Source: CAD feature listing. Evaluate the final solid. Frame: model axes, mm. Face numbers are marked on the shaded views. A direction names the side the tool comes from. Coordinates: 2 decimals unless noted, no trailing zeros. Order: outer loops, then holes, each group sorted by start corner. A loop starts at its lowest first (then second) coordinate and runs counter-clockwise, first axis right, second up. Notation, with made-up numbers: (-2.5, 29) - (3.5, 29) arc R16 cw to (3.5, 46) - close; hole circle Ø7 at (-12.5, 13). An arc over 180 degrees is marked (long way). One line per question, with ' | ' between items.
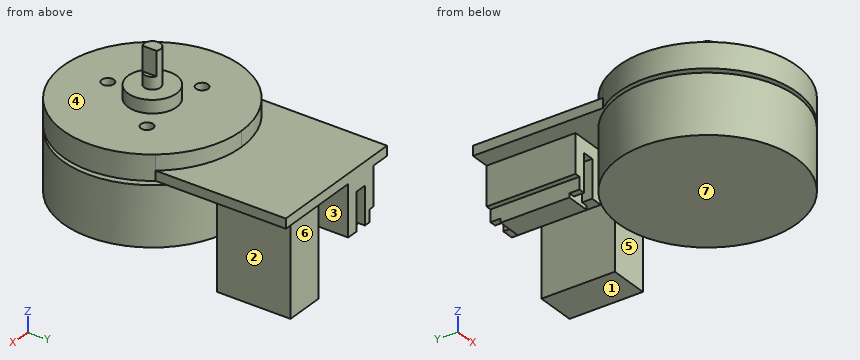
from build123d import *

# Parameters (mm, degrees)
SKETCH1_R           = 22
BOSS_EXTRUDE1_DEPTH = 21.83
SKETCH2_R           = 6
SKETCH2_R_2         = 2
BOSS_EXTRUDE2_DEPTH = 3.2
SKETCH3_R           = 2
BOSS_EXTRUDE3_DEPTH = 12.2
BOSS_EXTRUDE4_START = -6.2
BOSS_EXTRUDE4_DEPTH = 6.2
CUT_EXTRUDE3_START  = -3.8
CUT_EXTRUDE3_DEPTH  = 3.8
SKETCH7_W           = 9.7
SKETCH7_H           = 18.15
BOSS_EXTRUDE5_DEPTH = 26.4
SKETCH7_3_W         = 8.71
SKETCH7_3_H         = 22
BOSS_EXTRUDE6_DEPTH = 15
SKETCH8_R           = 1.5
CUT_EXTRUDE4_DEPTH  = 5
SKETCH9_W           = 1
SKETCH9_H           = 3.350814255
SKETCH10_W          = 6
SKETCH10_H          = 17
BOSS_EXTRUDE7_DEPTH = 1
SKETCH12_W          = 1.355
SKETCH12_H          = 22
CUT_EXTRUDE5_DEPTH  = 3
SKETCH13_W          = 2.841503492
SKETCH13_H          = 2.5
CUT_EXTRUDE6_DEPTH  = 9.35
CUT_EXTRUDE7_START  = -6
CUT_EXTRUDE7_DEPTH  = 6


with BuildPart() as part:
    # Sketch1 → Boss-Extrude1 (new body)
    with BuildSketch(Plane.XY):
        with Locations(Location((0, 0, 0), (0, 0, 180))):
            Circle(SKETCH1_R)
    extrude(amount=BOSS_EXTRUDE1_DEPTH)

    # Sketch2 → Boss-Extrude2 (add)
    with BuildSketch(Plane.XY.offset(21.83)):
        Circle(SKETCH2_R)
        Circle(SKETCH2_R_2, mode=Mode.SUBTRACT)
    extrude(amount=BOSS_EXTRUDE2_DEPTH)

    # Sketch3 → Boss-Extrude3 (add)
    with BuildSketch(Plane.XY.offset(21.83)):
        Circle(SKETCH3_R)
    extrude(amount=BOSS_EXTRUDE3_DEPTH)

    # Sketch4 → Boss-Extrude4 (add)
    with BuildSketch(Plane.XY.offset(21.83).offset(BOSS_EXTRUDE4_START)):
        Polygon((-17.5, 45.5), (-17.5, 22), (0, 22), (17.5, 22), (17.5, 45.5), align=None)
        with BuildLine():
            Line((0, 22), (-17.5, 22))
            Line((-17.5, 22), (-17.5, 13.332291626))
            ThreePointArc((-17.5, 13.332291626), (-9.764465787, 19.714340159), (0, 22))
        make_face()
        with BuildLine():
            Line((17.5, 22), (0, 22))
            ThreePointArc((0, 22), (9.764465787, 19.714340159), (17.5, 13.332291626))
            Line((17.5, 13.332291626), (17.5, 22))
        make_face()
    extrude(amount=BOSS_EXTRUDE4_DEPTH)

    # Sketch4_4 → Cut-Extrude3 (cut)
    with BuildSketch(Plane.XY.offset(21.83).offset(CUT_EXTRUDE3_START)):
        Polygon((-17.5, 45.5), (-17.5, 22), (0, 22), (17.5, 22), (17.5, 45.5), align=None)
        with BuildLine():
            Line((0, 22), (-17.5, 22))
            Line((-17.5, 22), (-17.5, 13.332291626))
            ThreePointArc((-17.5, 13.332291626), (-9.764465787, 19.714340159), (0, 22))
        make_face()
        with BuildLine():
            Line((17.5, 22), (0, 22))
            ThreePointArc((0, 22), (9.764465787, 19.714340159), (17.5, 13.332291626))
            Line((17.5, 13.332291626), (17.5, 22))
        make_face()
    extrude(amount=CUT_EXTRUDE3_DEPTH, mode=Mode.SUBTRACT)

    # Sketch7 → Boss-Extrude5 (add)
    with BuildSketch(Plane.XY.offset(18.03)):
        with Locations((8.23, 34.425)):
            Rectangle(SKETCH7_W, SKETCH7_H)
    extrude(amount=-BOSS_EXTRUDE5_DEPTH)

    # Sketch7_3 → Boss-Extrude6 (add)
    with BuildSketch(Plane.XY.offset(18.03)):
        with Locations((-8.445, 34.5)):
            Rectangle(SKETCH7_3_W, SKETCH7_3_H)
    extrude(amount=-BOSS_EXTRUDE6_DEPTH)

    # Sketch8 → Cut-Extrude4 (cut)
    with BuildSketch(Plane.XY.offset(21.83)):
        with Locations((-9.526279442, 5.5)):
            Circle(SKETCH8_R)
        with Locations((9.526279442, 5.5)):
            Circle(SKETCH8_R)
        with Locations((0, -11)):
            Circle(SKETCH8_R)
    extrude(amount=-CUT_EXTRUDE4_DEPTH, mode=Mode.SUBTRACT)

    # Sketch9 → Cut-Revolve1 (revolve, cut)
    with BuildSketch(Plane(origin=(0, 0, 0), x_dir=(0, 0, -1), z_dir=(1, 0, 0)), mode=Mode.PRIVATE) as cut_revolve1_sk:
        with Locations((-15.13, 20.324592872)):
            Rectangle(SKETCH9_W, SKETCH9_H)
    revolve(cut_revolve1_sk.sketch.rotate(Axis((0, 0, 34.03), (0, 0, -1)), 307.301790292), axis=Axis((0, 0, 34.03), (0, 0, -1)), mode=Mode.SUBTRACT)

    # Sketch10 → Boss-Extrude7 (add)
    with BuildSketch(Plane(origin=(0, 0, 3.03), x_dir=(-1, 0, 0), z_dir=(0, 0, -1))):
        with Locations((8.445, 34.5)):
            Rectangle(SKETCH10_W, SKETCH10_H)
    extrude(amount=BOSS_EXTRUDE7_DEPTH)

    # Sketch12 → Cut-Extrude5 (cut)
    with BuildSketch(Plane(origin=(0, 0, 3.03), x_dir=(-1, 0, 0), z_dir=(0, 0, -1))):
        with Locations((12.1225, 34.5)):
            Rectangle(SKETCH12_W, SKETCH12_H)
    extrude(amount=-CUT_EXTRUDE5_DEPTH, mode=Mode.SUBTRACT)

    # Sketch13 → Cut-Extrude6 (cut)
    with BuildSketch(Plane(origin=(0, 0, 3.03), x_dir=(-1, 0, 0), z_dir=(0, 0, -1))):
        with Locations((8.445, 44.25)):
            Rectangle(SKETCH13_W, SKETCH13_H)
        with Locations((8.445, 24.75)):
            Rectangle(SKETCH13_W, SKETCH13_H)
    extrude(amount=-CUT_EXTRUDE6_DEPTH, mode=Mode.SUBTRACT)

    # Sketch14 → Cut-Extrude7 (cut)
    with BuildSketch(Plane.XY.offset(34.03).offset(CUT_EXTRUDE7_START)):
        with BuildLine():
            Line((1, 1.732050808), (1, -1.732050808))
            ThreePointArc((1, -1.732050808), (2, 0), (1, 1.732050808))
        make_face()
    extrude(amount=CUT_EXTRUDE7_DEPTH, mode=Mode.SUBTRACT)


solid = part.part
(1) Pull-direction query (X, two-part tool) for the marked faces 1, 2 and 3; classes: pulls with the +X half, pulls with the -X half, needs draft (parallel to the pull), parting line crosses it, or undercut.
Taken from the geometry:
face 1: needs draft | face 2: pulls with the +X half | face 3: undercut
(2) Set-up query: the marked faces 4, 5, 6 and 7. Return all of +Z, -Z, +X, -X, +Y, -Y with unobstructed straight access to the full face (end or side cutting, diameter ignored); none if empty.
Taken from the geometry:
face 4: +Z | face 5: -Z, +X | face 6: -Z, +X, +Y | face 7: -Z, +X, -X, -Y
(3) Material intervals for L1, parallel to X at y = 31, z = 3.5 (3 decimals); L2, parallel to Z at x = 16.5, y = 10.5; L3, parallel to X at y = 5, z = 20, sorted ascending. Write a range as from..to.
Taken from the geometry:
L1: x = -11.445..-4.09, 3.38..13.08 | L2: z = 0..14.63, 15.63..21.83 | L3: x = -21.42..-10.94, -8.11..8.11, 10.94..21.42
(4) Cut plane B-B (y = 0). Return the cut outline in (x, z), and give its area (3 significant figures).
Taken from the geometry:
outline: (-22, 0) - (22, 0) - (22, 14.63) - (18.65, 14.63) - (18.65, 15.63) - (22, 15.63) - (22, 21.83) - (6, 21.83) - (6, 25.03) - (2, 25.03) - (2, 28.03) - (1, 28.03) - (1, 34.03) - (-2, 34.03) - (-2, 25.03) - (-6, 25.03) - (-6, 21.83) - (-22, 21.83) - (-22, 15.63) - (-18.65, 15.63) - (-18.65, 14.63) - (-22, 14.63) - close | area: 1,020 mm²
(5) Cut plane C-C (z = 19.5). Return the cut outline in (x, y).
Taken from the geometry:
outline: circle Ø44 at (0, 0); hole circle Ø3 at (-9.53, 5.5); hole circle Ø3 at (0, -11); hole circle Ø3 at (9.53, 5.5)
(6) Cut plane D-D (y = 30). Return the cut outline in (x, z) (3 decimals), and give its area (3 significant figures).
Taken from the geometry:
outline: (-17.5, 15.63) - (-12.8, 15.63) - (-12.8, 6.03) - (-11.445, 6.03) - (-11.445, 2.03) - (-5.445, 2.03) - (-5.445, 3.03) - (-4.09, 3.03) - (-4.09, 15.63) - (3.38, 15.63) - (3.38, -8.37) - (13.08, -8.37) - (13.08, 15.63) - (17.5, 15.63) - (17.5, 18.03) - (-17.5, 18.03) - close | area: 428 mm²
(7) Pin query (flat end, axial travel): P1, Ø14.5, axis at y = 38.5, z = 0, coming from the -X side; P2, Ø10, axis at y = 30, z = 8, coming from the +X side; P3, Ø10, axis at x = 9.5, y = -4, coming from the -Z side. Return the tip coordinate at first contact, or that it passes through.
Taken from the geometry:
P1: stops at x = -12.8 | P2: stops at x = 13.08 | P3: stops at z = 0
(8) Cut plane A-A (z = 11). Return the cut outline in (x, y).
Taken from the geometry:
outline: circle Ø44 at (0, 0); (-12.8, 23.5) - (-9.87, 23.5) - (-9.87, 26) - (-7.02, 26) - (-7.02, 23.5) - (-4.09, 23.5) - (-4.09, 45.5) - (-7.02, 45.5) - (-7.02, 43) - (-9.87, 43) - (-9.87, 45.5) - (-12.8, 45.5) - close; (3.38, 25.35) - (13.08, 25.35) - (13.08, 43.5) - (3.38, 43.5) - close
